The figure shows three views and two pictorial views of one solid part (mm, origin at its lowest corner). Answer the questions. A direction names the side the tool comes from. Give positions to 0.01 mm unless a question says otherwise; leave off trailing zeros. Order: outer loops, then holes, each group sorted by start corner. A loop starts at its lowest first (then second) coordinate and runs counter-clockwise, first axis right, second up. Notation, with made-up numbers: M 45,25.25 L 55,25.25 A27 ccw 55,50.25 Z; hole C 84.25,10.25 d4. An arc over 180 degrees is marked long. One line per item, written item: value. Start each with the question number.
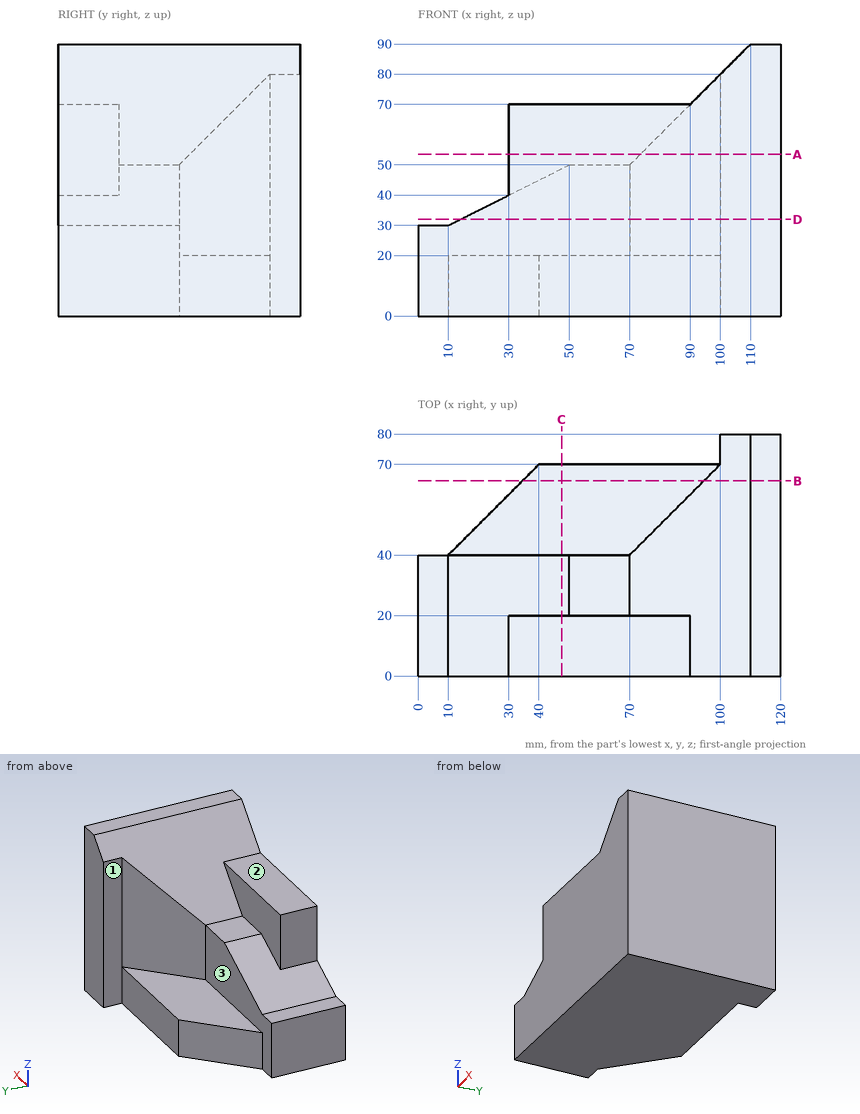
Q1. Find section D-D, the plane z = 32. Give the vertices of the cut face in (x, y).
Q2. Find section A-A, the plane z = 53.5. Give the vertices of the cut face in (x, y).
Q3. Consider probe 1 along X at (y, z) = (10, 66); probe 2 along Y at (x, z) = (41.5, 59.5); probe 3 along X at (y, z) = (50, 57.5). Determine where each line is inside the solid, lowest interval first.
Q4. Each of these flat-tipped pins is pushed along its axis until it touches: pin 1 (6 mm diameter, centred on y = 6.5, z = 57, fed in from -X); pin 2 (10 mm diameter, centred on y = 21.5, z = 26.5, fed in from -X); pin 3 (16 mm diameter, centred on x = 67, z = 11.5, fed in from +Y); pin 4 (6 mm diameter, centred on x = 44, z = 32.5, fed in from +Y). Where does it stop, or does it pass through?
Q5. Find section B-B, the plane y = 64.5. Give the vertices of the cut face in (x, z), then the cut area to 3 significant figures.
Q6. Find section C-C, the plane x = 47.5. Give the vertices of the cut face in (y, z).
Q7. A tool of negligible diameter and unlimited length cuts with its end or side. For the marked faces 1, 2 and 3, from which of +Z, -Z, +X, -X, +Y, -Y can it reach the whole face along a straight path? Write none if from no direction.
Evaluation:
1. outline: M 14,0 L 120,0 L 120,80 L 100,80 L 100,70 L 70,40 L 14,40 Z
2. outline: M 30,0 L 120,0 L 120,80 L 100,80 L 100,70 L 73.5,43.5 L 73.5,20 L 30,20 Z
3. probe 1: 30 to 120
3. probe 2: 0 to 20
3. probe 3: 80 to 120
4. pin 1: x = 30
4. pin 2: x = 0
4. pin 3: y = 70
4. pin 4: y = 40
5. outline: M 34.5,0 L 120,0 L 120,90 L 110,90 L 94.5,74.5 L 94.5,20 L 34.5,20 Z
5. area: 3,370 mm2
6. outline: M 0,0 L 70,0 L 70,20 L 40,20 L 40,48.75 L 20,48.75 L 20,70 L 0,70 Z
7. face 1: +Z, -Z, -X, +Y
7. face 2: +Z, -X, +Y, -Y
7. face 3: +Z, -X, +Y
